```python
from build123d import *

# Parameters (mm, degrees)
PAD008_DEPTH    = 40
POCKET006_DEPTH = 40
POCKET007_DEPTH = 40
SKETCH014_R     = 2.1
POCKET008_DEPTH = 25.001


with BuildPart() as part:
    # Sketch011 → Pad008 (new body)
    with BuildSketch(Plane.XY):
        with BuildLine():
            ThreePointArc((24.9048674523, 2.1788935687), (0, 25), (-24.9048674523, 2.1788935687))
            ThreePointArc((-24.9048674523, 2.1788935687), (-24.620193675, 0.0165817754), (-24.1481451973, -2.1126907965))
            Line((-24.1481451973, -2.1126907965), (24.148145198, -2.1126907965))
            ThreePointArc((24.148145198, -2.1126907965), (24.6201936752, 0.0165817755), (24.9048674523, 2.1788935687))
        make_face()
    extrude(amount=PAD008_DEPTH)

    # Sketch012 → Pocket006 (cut)
    with BuildSketch(Plane.XY):
        with BuildLine():
            ThreePointArc((22.909479324, 2.0385674149), (0, 23), (-22.909479324, 2.0385674149))
            Line((-22.909479324, 2.0385674149), (22.909479324, 2.0385674149))
        make_face()
    extrude(amount=POCKET006_DEPTH, mode=Mode.SUBTRACT)

    # Sketch013 → Pocket007 (cut)
    with BuildSketch(Plane.XY):
        with BuildLine():
            ThreePointArc((-22.912478289, 2.3532080284), (3.93e-08, -18.642213), (22.9124783677, 2.3532080284))
            Line((-22.912478289, 2.3532080284), (22.9124783677, 2.3532080284))
        make_face()
    extrude(amount=POCKET007_DEPTH, mode=Mode.SUBTRACT)

    # Sketch014 → Pocket008 (cut, through all)
    with BuildSketch(Plane.XZ):
        with Locations((0, 20.063227)):
            Circle(SKETCH014_R)
    extrude(amount=-POCKET008_DEPTH, mode=Mode.SUBTRACT)


solid = part.part
```
The model under review builds one solid part; all positions refer to its coordinate system, in mm. A direction names the side the tool comes from. Coordinates: 2 decimals unless noted, no trailing zeros. Write each loop counter-clockwise with the first axis right and the second up, starting at its lowest first coordinate (ties: lowest second). Pieces come first, ordered by that corner, then holes. Notation, with made-up numbers: (60.5, -11) - (80.5, -11) arc R23 cw to (80.5, 3) - close; hole circle Ø7 at (-16.75, 60.5). An arc over 180 degrees is marked (long way). Answer in a Markdown table with one row per item. Add a question column.
Q1. Consider section D-D on x = -21.5. Give the boundary of the cut face in (y, z).
Q2. Clearance check with flat-ended pins moving along their axes: pin 1 (1.5 mm diameter, centred on x = -10, z = 12.5, fed in from +Y); pin 2 (5 mm diameter, centred on x = 4.5, z = 27.5, fed in from -Y); pin 3 (12 mm diameter, centred on y = 21, z = 29.5, fed in from -X). State where each tip first meets the part, or that it passes through.
Q3. To check wall thickness, follow line 1 along Z through (x, y) = (0, 23.8); line 2 along X through (y, z) = (17.75, 27); line 3 along X through (y, z) = (21.25, 5). State the ranges of each line that lie inside material, in increasing order. Write a range as from..to.
Q4. Consider section B-B on y = 18.75. Give the boundary of the cut face in (x, z), then the cut area to 3 significant figures.
Q5. Consider section A-A on x = 0. Give the boundary of the cut face in (y, z), then the cut area to 3 significant figures.
Q6. For faces 1 (the face through (22.567, -0.085, 19.72)), 2 (the face through (23, -2.113, 20)), list the 3-axis set-ups (+Z, -Z, +X, -X, +Y, -Y) from which the entire face can be reached by the end or side of a thin tool; tool diameter is ignored.
Q7. Draft analysis for pull direction Y (two halves, no side actions). For faces 3 (the face through (-22.578, -0.027, 19.72)), 4 (the face through (0.519, 24.995, 24.164)), 5 (the face through (-23, -2.113, 20)), state which applies: +Y half, -Y half, draft (parallel to the pull), parting line (faces both ways), or undercut.
Answers below:
| question | item | result |
|---|---|---|
| 1 | outline | (8.17, 0) - (12.76, 0) - (12.76, 40) - (8.17, 40) - close |
| 2 | pin 1 | y = 23.23 |
| 2 | pin 2 | y = 21.91 |
| 2 | pin 3 | x = -20 |
| 3 | line 1 | 0..17.96, 22.16..40 |
| 3 | line 2 | -17.61..-14.63, 14.63..17.61 |
| 3 | line 3 | -13.17..-8.8, 8.8..13.17 |
| 4 | outline | (-16.54, 0) - (-13.32, 0) - (-13.32, 40) - (-16.54, 40) - close; (13.32, 0) - (16.54, 0) - (16.54, 40) - (13.32, 40) - close |
| 4 | area | 257 mm² |
| 5 | outline | (23, 0) - (25, 0) - (25, 17.96) - (23, 17.96) - close; (23, 22.16) - (25, 22.16) - (25, 40) - (23, 40) - close |
| 5 | area | 71.6 mm² |
| 6 | face 1 | +Z, -Z |
| 6 | face 2 | +Z, -Z, +X, -X, -Y |
| 7 | face 3 | undercut |
| 7 | face 4 | +Y half |
| 7 | face 5 | -Y half |
